The model under review builds one solid part; all positions refer to its coordinate system, in mm. A direction names the side the tool comes from. Give positions to 0.01 mm unless a question says otherwise; leave off trailing zeros. Loops run counter-clockwise (first coordinate to the right, second up) from the corner with the lowest first, then second, coordinate; pieces in that order, holes last. Notation, with made-up numbers: M 27.5,13.5 L 42.5,13.5 A24 ccw 42.5,24.5 Z; hole C 7.5,68.25 d4. An arc over 180 degrees is marked long. Write item = value, one per line. Start each with the question number.
1. Draft analysis for pull direction X (two halves, no side actions). For faces 5 (the face through (0.659, -2.958, -1.207)), 6 (the face through (-1.79, -43.35, -3.3)), 7 (the face through (3, -35.5, 3)), state which applies: pulls with the +X half, pulls with the -X half, needs draft (parallel to the pull), parting line crosses it, or undercut.
2. For faces 1 (the face through (-1.979, -39.198, 3.358)), 2 (the face through (1.979, -39.198, -3.358)), 3 (the face through (2.285, -16.269, 3.584)), 4 (the face through (1.92, -39.2, 3.39)), list the 3-axis set-ups (+Z, -Z, +X, -X, +Y, -Y) from which the entire face can be reached by the end or side of a thin tool; tool diameter is ignored.
3. We need section A-A on y = -3. Give the boundary of the cut face in (x, z) (3 decimals).
4. We need section B-B on y = -8. Give the boundary of the cut face in (x, z).
5. Wall thickness on line 1 along Y through (x, z) = (1.25, -6); line 2 along Y through (x, z) = (0.75, 1); line 3 along Z through (x, y) = (2.5, -10): over which ranges is each line inside the solid? List them lowest first. Write a range as from..to.
6. For pin 1 (1 mm diameter, centred on x = -6, z = -1.5, fed in from -Y); pin 2 (5 mm diameter, centred on y = -34.5, z = -0.5, fed in from -X); pin 3 (1 mm diameter, centred on x = 1.5, z = -4, fed in from -Y); pin 4 (4 mm diameter, centred on x = -1, y = -26.5, fed in from -Z), all flat-tipped, find the tip position at first contact; note any pin that passes through.
from build123d import *

# Parameters (mm, degrees)
F0_R     = 4.25
F1_DEPTH = 33
F2_DEPTH = 6
F3_R     = 7.5
F3_R_2   = 4.25
F4_DEPTH = 2.5
F6_DEPTH = 8
F7_R     = 0.5
F8_R     = 1


with BuildPart() as f1:
    # F0 (on Front) → F1 (new body)
    with BuildSketch(Plane.XZ):
        Circle(F0_R)
        Polygon((-1.375, 2.38157), (2.75, 0), (-1.375, -2.38157), align=None, mode=Mode.SUBTRACT)
        Polygon((-1.375, -2.38157), (2.75, 0), (-1.375, 2.38157), align=None)
    extrude(amount=F1_DEPTH)

    # F0 (on Front) → F2 (cut)
    with BuildSketch(Plane.XZ):
        Polygon((-1.375, -2.38157), (2.75, 0), (-1.375, 2.38157), align=None)
    extrude(amount=F2_DEPTH, mode=Mode.SUBTRACT)

    # F3 (on face) → F4 (join)
    with BuildSketch(Plane.XZ.offset(33)):
        Circle(F3_R)
        Circle(F3_R_2, mode=Mode.SUBTRACT)
        Circle(F3_R_2)
    extrude(amount=F4_DEPTH)

    # F5 (on face) → F6 (join)
    with BuildSketch(Plane.XZ.offset(35.5)):
        Polygon((0.076423, -4.499351), (3.934764, -2.183492), (3.858341, 2.315859), (-0.076423, 4.499351), (-3.934764, 2.183492), (-3.858341, -2.315859), align=None)
    extrude(amount=F6_DEPTH)

    # F7
    f7_edges = [f1.edges().sort_by_distance(p)[0] for p in [
        (2.005593, -43.5, -3.341421),
        (-1.890959, -43.5, -3.407605),
        (-3.896552, -43.5, -0.066184),
        (-2.005593, -43.5, 3.341421),
        (1.890959, -43.5, 3.407605),
        (3.896552, -43.5, 0.066184),
    ]]
    fillet(f7_edges, radius=F7_R)

    # F8
    f8_edges = [f1.edges().sort_by_distance(p)[0] for p in [
        (-7.5, -35.5, 0),
        (-7.5, -33, 0),
    ]]
    fillet(f8_edges, radius=F8_R)


solid = f1.part
Final values:
q1.face_5 = undercut
q1.face_6 = pulls with the -X half
q1.face_7 = needs draft
q2.face_1 = +Z, -X, -Y
q2.face_2 = -Z, +X, -Y
q2.face_3 = +Y
q2.face_4 = +Z, +X, -Y
q3.outline = C 0,0 d8.5; hole M -1.375,-2.382 L 2.75,0 L -1.375,2.382 Z
q4.outline = C 0,0 d8.5
q5.line_1 = -35.5..-33
q5.line_2 = -43.5..-6
q5.line_3 = -3.44..3.44
q6.pin_1 = -35.5
q6.pin_2 = -7.5
q6.pin_3 = -43.4
q6.pin_4 = -4.25
